The listing builds one solid part. Answer for the finished solid, in the listing's coordinates (mm). A direction names the side the tool comes from. Round coordinates to 2 decimals unless told otherwise and drop trailing zeros. Loops run counter-clockwise (first coordinate to the right, second up) from the corner with the lowest first, then second, coordinate; pieces in that order, holes last. Notation, with made-up numbers: (5.25, 33) - (10.25, 33) arc R27 cw to (10.25, 56) - close; hole circle Ø3 at (-15, 64.5). An arc over 180 degrees is marked (long way). Write item = value, one per line. Start each with the question number.
1) Section A-A, the plane z = 0 is taken. Determine the outline of the cut face in (x, y) (1 decimal), and give its area (3 significant figures).
2) A tool of negligible diameter and unlimited length cuts with its end or side. For faces 5 (the flat face through (18.225, -5.344, -10.058)), 6 (the flat face through (16.408, -1, 8)), 7 (the flat face through (18.694, 0, 0)), 8 (the flat face through (9, -4, -8.255)), 9 (the cylindrical face through (6.52, -3.51, 9.94)), from which of +Z, -Z, +X, -X, +Y, -Y can it reach the whole face along a straight path? Write none if from no direction.
3) Straight lines are drawn through the part: line 1 along X through (y, z) = (-3, -1.5); line 2 along Z through (x, y) = (16, -0.5) (1 decimal); line 3 along X through (y, z) = (-5.5, 7). For each, find the intervals that lie inside material, in ascending order.
4) For a pull along Y with two mould halves and no side action, classify faces 1 (the flat face through (15.506, 0, 8)), 2 (the flat face through (2.286, 0, -2)), 3 (the flat face through (12.38, -5.36, 7.17)), 4 (the cylindrical face through (9.23, 9.824, -3.822)) as released by +Y, released by -Y, zero draft, split by the parting line, or undercut.
5) Section B-B, the plane x = 9 is taken. Determine the outline of the cut face in (y, z) (1 decimal).
6) Section D-D, the plane x = 6.25 is taken. Determine the outline of the cut face in (y, z) (1 decimal), and give its area (3 significant figures).
7) Section C-C, the plane y = -5.25 is taken. Determine the outline of the cut face in (x, z) (1 decimal).
8) Given pin 1 Ø1.5 at (y, z) = (-4, 7.5) entering from -X; pin 2 Ø3.5 at (x, z) = (10, -4) entering from +Y; pin 3 Ø2.5 at (x, y) = (10.5, -5.5) entering from +Z; pin 4 Ø5 at (x, z) = (10, -6.5) entering from +Y, each flat-ended and moving along its own axis, determine where each tip first touches the part or whether it passes through.
from build123d import *

# Parameters (mm, degrees)
BOSS_EXTRUDE1_DEPTH      = 18.6944
CHAMFER1_SIZE            = 0.9525
SKETCH2_W                = 14.1224
SKETCH2_H                = 18.796
CUT_EXTRUDE1_DEPTH       = 6.35
SHELL2_START             = 2.286
SHELL2_DEPTH             = 14.1224
BOSS_EXTRUDE3_REACH      = 28.031
BOSS_EXTRUDE3_END_RADIUS = 10.541
BOSS_EXTRUDE4_DEPTH      = 1.27
BOSS_EXTRUDE4_DEPTH_BACK = 0.9525
SKETCH4_W                = 14.473113765
SKETCH4_H                = 19.407327032


# Read off the part's stored shape, not the designer's step: Shell2
with BuildPart() as part:
    # Sketch1 → Boss-Extrude1 (new body)
    with BuildSketch(Plane(origin=(0, 0, 0), x_dir=(0, 0, -1), z_dir=(1, 0, 0))):
        with BuildLine():
            Line((-10.541, 0), (-10.541, -10.541))
            Line((-10.541, -10.541), (10.541, -10.541))
            Line((10.541, -10.541), (10.541, 0))
            ThreePointArc((10.541, 0), (0, 10.541), (-10.541, 0))
        make_face()
    extrude(amount=BOSS_EXTRUDE1_DEPTH)

    # Chamfer1
    chamfer1_edges = [part.edges().sort_by_distance(p)[0] for p in [
        (18.6944, -5.2705, 10.541),
        (18.6944, -5.2705, -10.541),
        (0, -5.2705, 10.541),
        (0, 10.541, 0),
        (0, -5.2705, -10.541),
        (18.6944, 10.541, 0),
    ]]
    chamfer(chamfer1_edges, length=CHAMFER1_SIZE)

    # Sketch2 → Cut-Extrude1 (cut)
    with BuildSketch(Plane.XY.offset(10.541)):
        with Locations((9.3472, -1.143)):
            Rectangle(SKETCH2_W, SKETCH2_H)
    extrude(amount=-CUT_EXTRUDE1_DEPTH, mode=Mode.SUBTRACT)

    # Shell2 outline → Shell2 (cut)
    with BuildSketch(Plane.YZ.offset(SHELL2_START)):
        with BuildLine():
            ThreePointArc((0, -8.255), (7.167347138, -4.095626936), (7.112, 4.191))
            Line((7.112, 4.191), (-8.255, 4.191))
            Line((-8.255, 4.191), (-8.255, -8.255))
            Line((-8.255, -8.255), (0, -8.255))
        make_face()
    extrude(amount=SHELL2_DEPTH, mode=Mode.SUBTRACT)



with BuildPart() as body_2:
    # Boss-Extrude3: up to this cylinder (the profile starts inside it)
    boss_extrude3_end = Plane(origin=(6.361697, 0, 0), z_dir=(-1, 0, 0)) * Cylinder(BOSS_EXTRUDE3_END_RADIUS, 78.144, mode=Mode.PRIVATE)
    # Sketch3 → Boss-Extrude3 (new, up to the surface)
    with BuildSketch(Plane.XY.offset(4.191), mode=Mode.PRIVATE) as boss_extrude3_sk1:
        Polygon((9.3472, 7.112), (3.188027328, 3.556), (3.188027328, -3.556), (9.3472, -7.112), (15.506372672, -3.556), (15.506372672, 3.556), align=None)
        Polygon((9.3472, 4.765648506), (5.220027328, 2.382824253), (5.220027328, -2.382824253), (9.3472, -4.765648506), (13.474372672, -2.382824253), (13.474372672, 2.382824253), align=None, mode=Mode.SUBTRACT)
    boss_extrude3_tool1 = extrude(boss_extrude3_sk1.sketch, amount=BOSS_EXTRUDE3_REACH, mode=Mode.PRIVATE) & boss_extrude3_end
    add(boss_extrude3_tool1.solids().sort_by_distance((6.361697, 5.171044, 4.191))[0])


with BuildPart() as part_1:
    add(part.part)

    add(body_2.part)  # Boss-Extrude4 merges body 2
    # Sketch4 → Boss-Extrude4 (add, two sides: drawn at the far end of the back side and taken through both)
    with BuildSketch(Plane.XY.offset(4.191).offset(-BOSS_EXTRUDE4_DEPTH_BACK)):
        with Locations((9.522556883, -0.837336484)):
            Rectangle(SKETCH4_W, SKETCH4_H)
    extrude(amount=BOSS_EXTRUDE4_DEPTH + BOSS_EXTRUDE4_DEPTH_BACK)


solid = part_1.part
Geometry check:
q1.outline = (0, -10.5) - (18.7, -10.5) - (18.7, 9.6) - (17.7, 10.5) - (1, 10.5) - (0, 9.6) - close; hole (2.3, -8.3) - (16.4, -8.3) - (16.4, 8.3) - (2.3, 8.3) - close
q1.area = 160 mm2
q2.face_5 = -Z, +X, +Y, -Y
q2.face_6 = +Z, -Y
q2.face_7 = +Z, -Z, +X, +Y, -Y
q2.face_8 = none
q2.face_9 = +Z
q3.line_1 = 0 to 2.29, 16.41 to 18.69
q3.line_2 = -10.5 to -8.3, 3.2 to 5.5
q3.line_3 = 0 to 2.29, 6.56 to 12.14, 16.41 to 18.69
q4.face_1 = zero draft
q4.face_2 = undercut
q4.face_3 = released by -Y
q4.face_4 = released by +Y
q5.outline = (-10.5, -10.5) - (0, -10.5) arc R10.5 ccw to (8.3, 6.6) - (8.3, 5.5) - (6.9, 5.5) - (6.9, 8) arc R10.5 ccw to (4.6, 9.5) - (4.6, 5.5) - (-4.6, 5.5) - (-4.6, 9.5) arc R10.5 ccw to (-6.9, 8) - (-6.9, 5.5) - (-10.5, 5.5) - close; hole (-8.3, -8.3) - (0, -8.3) arc R8.3 ccw to (7.6, 3.2) - (-8.3, 3.2) - close
q6.outline = (-10.5, -10.5) - (0, -10.5) arc R10.5 ccw to (8.3, 6.6) - (8.3, 5.5) - (5.3, 5.5) - (5.3, 9.1) arc R10.5 ccw to (3, 10.1) - (3, 5.5) - (-3, 5.5) - (-3, 10.1) arc R10.5 ccw to (-5.3, 9.1) - (-5.3, 5.5) - (-10.5, 5.5) - close; hole (-8.3, -8.3) - (0, -8.3) arc R8.3 ccw to (7.6, 3.2) - (-8.3, 3.2) - close
q6.area = 157 mm2
q7.outline = (0, -9.6) - (1, -10.5) - (17.7, -10.5) - (18.7, -9.6) - (18.7, 9.6) - (17.7, 10.5) - (16.4, 10.5) - (16.4, 5.5) - (12.6, 5.5) - (12.6, 9.1) - (6.1, 9.1) - (6.1, 5.5) - (2.3, 5.5) - (2.3, 10.5) - (1, 10.5) - (0, 9.6) - close; hole (2.3, -8.3) - (16.4, -8.3) - (16.4, 3.2) - (2.3, 3.2) - close
q8.pin_1 = 0
q8.pin_2 = 10.3
q8.pin_3 = 9.65
q8.pin_4 = 9.75
